from build123d import *

# Parameters (mm, degrees)
F0_R      = 10.289099
F2_DEPTH  = 26.4
F4_R      = 5
F5_R      = 5.460042
F3_R      = 5.477672
F6_DEPTH  = 10.3
F7_R      = 2.997671
F8_DEPTH  = 15.6
F9_R      = 3.220939
F10_DEPTH = 25
F11_R     = 5.627011
F12_DEPTH = 29.6
F13_R     = 5.708665
F14_DEPTH = 6.4
F15_R     = 4.005465
F16_DEPTH = 46.1
F18_DEPTH = 44.9


with BuildPart() as f2:
    # F0 (on Front) → F2 (new body)
    with BuildSketch(Plane.XZ):
        Circle(F0_R)
    extrude(amount=F2_DEPTH)

    # F4
    f4_edges = [f2.edges().sort_by_distance(p)[0] for p in [
        (-10.289099, -26.4, 0),
        (-10.289099, 0, 0),
    ]]
    fillet(f4_edges, radius=F4_R)

    # F5 (on Front) + F3 (on Front) → F6 (cut)
    with BuildSketch(Plane.XZ):
        Circle(F5_R)
    with BuildSketch(Plane.XZ):
        Circle(F3_R)
    extrude(amount=F6_DEPTH, mode=Mode.SUBTRACT)

    # F7 (on Top) → F8 (cut)
    with BuildSketch(Plane.XY):
        with Locations((4.320451, -17.085413)):
            Circle(F7_R)
    extrude(amount=-F8_DEPTH, mode=Mode.SUBTRACT)

    # F9 (on Top) → F10 (cut)
    with BuildSketch(Plane.XY):
        with Locations((-4.516833, -17.674565)):
            Circle(F9_R)
    extrude(amount=-F10_DEPTH, mode=Mode.SUBTRACT)

    # F11 (on Front) → F12 (join)
    with BuildSketch(Plane.XZ):
        Circle(F11_R)
    extrude(amount=F12_DEPTH)

    # F13 (on Front) → F14 (cut)
    with BuildSketch(Plane.XZ):
        Circle(F13_R)
    extrude(amount=F14_DEPTH, mode=Mode.SUBTRACT)

    # F15 (on Front) → F16 (cut, symmetric)
    with BuildSketch(Plane.XZ):
        Circle(F15_R)
    extrude(amount=F16_DEPTH, both=True, mode=Mode.SUBTRACT)

    # F17 (on Top) → F18 (cut)
    with BuildSketch(Plane.XY):
        with BuildLine():
            ThreePointArc((-3.731297, -9.23005), (-0.012911, -8.641232), (3.731297, -9.033666))
            ThreePointArc((3.731297, -9.033666), (-0.061388, -6.799126), (-3.731297, -9.23005))
        make_face()
    extrude(amount=-F18_DEPTH, mode=Mode.SUBTRACT)


solid = f2.part
Source: CAD feature listing. Evaluate the final solid. Frame: model axes, mm. A direction names the side the tool comes from. Coordinates: 2 decimals unless noted, no trailing zeros. Order: outer loops, then holes, each group sorted by start corner. A loop starts at its lowest first (then second) coordinate and runs counter-clockwise, first axis right, second up.
Item 1: Cut plane B-B (z = -0.5). Count the separate pieces of the cut face and the enclosed holes in it, plus the area to 3 significant figures.
Output values:
separate pieces: 2
enclosed holes: 2
area: 284 mm2
Item 2: Material intervals for line 1 (Y direction, x = 1, z = -4); line 2 (Y direction, x = -5, z = 2.5); line 3 (Z direction, x = -4, y = -1.5), sorted ascending.
Output values:
line 1: y = -29.6 to -8.65, -6.91 to -6.4
line 2: y = -29.6 to -6.4
line 3: z = -7.91 to -4.07, 4.07 to 7.91
Item 3: First-contact query: P1, Ø4, axis at y = -3.5, z = 6, coming from the +X side; P2, Ø5, axis at x = 5.5, y = -20.5, coming from the +Z side; P3, Ø3.5, axis at x = 0.5, z = 1.5, coming from the +Y side; P4, Ø1, axis at x = -2.5, y = -19.5, coming from the +Z side. Flat tips, straight axial feed; report the tip coordinate or a pass-through.
Output values:
P1: stops at x = 9.36
P2: stops at z = 9.84
P3: passes through
P4: stops at z = 10.09
Item 4: Pull-direction query (X, two-part tool) for faces 4 (the face through (4, -29.6, -2)), 5 (the face through (5.445, -3.164, 1.715)), 6 (the face through (-1.34, -13.09, 10.2)); classes: pulls with the +X half, pulls with the -X half, needs draft (parallel to the pull), parting line crosses it, or undercut.
Output values:
face 4: needs draft
face 5: undercut
face 6: parting line crosses it
Item 5: Cut plane A-A (x = 0). Return loops of the section in (y, z), plus the area to 3 significant figures.
Output values:
outline: (-29.6, -5.63) - (-26.39, -5.63) arc R5 ccw to (-21.4, -10.29) - (-8.64, -10.29) - (-8.64, -4.01) - (-29.6, -4.01) - close; (-29.6, 4.01) - (-6.4, 4.01) - (-6.4, 5.71) - (-0.02, 5.71) arc R5 ccw to (-5, 10.29) - (-21.4, 10.29) arc R5 ccw to (-26.39, 5.63) - (-29.6, 5.63) - close; (-6.8, -10.29) - (-5, -10.29) arc R5 ccw to (-0.02, -5.71) - (-6.4, -5.71) - (-6.4, -4.01) - (-6.8, -4.01) - close
area: 287 mm2
Item 6: Set-up query: faces 1 (the face through (2, -6.4, -4)), 2 (the face through (4.39, -17.04, -3.52)), 3 (the face through (5.198, -27.972, -2.155)). Return all of +Z, -Z, +X, -X, +Y, -Y with unobstructed straight access to the full face (end or side cutting, diameter ignored); none if empty.
Output values:
face 1: +Y
face 2: -Z
face 3: -Y
Item 7: Cut plane C-C (y = -13). Return loops of the section in (x, z), plus the area to 3 significant figures.
Output values:
outline: circle Ø20.58 at (0, 0); hole circle Ø8.01 at (0, 0)
area: 282 mm2
